from build123d import *

# Parameters (mm, degrees)
F0_W     = 33
F0_H     = 15
F1_DEPTH = 12
F2_W     = 31.2
F2_H     = 12.2
F3_DEPTH = 10
F4_W     = 30
F4_H     = 11
F5_DEPTH = 12.001


with BuildPart() as f1:
    # F0 (on Top) → F1 (new body)
    with BuildSketch(Plane.XY):
        with Locations((16.5, 7.5)):
            Rectangle(F0_W, F0_H)
    extrude(amount=F1_DEPTH)

    # F2 (on face) → F3 (cut)
    with BuildSketch(Plane.XY.offset(12)):
        with Locations((16.5, 7.5)):
            Rectangle(F2_W, F2_H)
    extrude(amount=-F3_DEPTH, mode=Mode.SUBTRACT)

    # F4 (on face) → F5 (cut, through all)
    with BuildSketch(Plane(origin=(0, 0, 0), x_dir=(1, 0, 0), z_dir=(0, 0, -1))):
        with Locations((16.5, -7.5)):
            Rectangle(F4_W, F4_H)
    extrude(amount=-F5_DEPTH, mode=Mode.SUBTRACT)


solid = f1.part
The model under review builds one solid part; all positions refer to its coordinate system, in mm. A direction names the side the tool comes from. Coordinates: 2 decimals unless noted, no trailing zeros. Write each loop counter-clockwise with the first axis right and the second up, starting at its lowest first coordinate (ties: lowest second). Pieces come first, ordered by that corner, then holes. Notation, with made-up numbers: (75.5, 52.5) - (106.5, 52.5) arc R25 cw to (106.5, 70.5) - close; hole circle Ø3 at (41.25, 68). An arc over 180 degrees is marked (long way). Answer as a JSON object with one key per item and string values. Group by question number.
1. Mouldability with a two-part tool opening along X and no side actions: class faces 1 (the face through (16, 13.6, 7)), 2 (the face through (18, 14, 12)), 3 (the face through (0, 7, 6)) as pulls with the +X half, pulls with the -X half, needs draft (parallel to the pull), parting line crosses it, or undercut.
2. Machinability: for faces 4 (the face through (16, 13, 1)), 5 (the face through (16, 0, 6)), 6 (the face through (32.1, 7, 7)), which of the approach directions +Z, -Z, +X, -X, +Y, -Y give a long, thin tool a straight path to every point of the face, cutting with its end or side? Answer none if there is none.
3. Add section B-B (y = 6.5). Give the boundary of the cut face in (x, z), plus the area to 3 significant figures.
4. Add section A-A (z = 3). Give the boundary of the cut face in (x, y).
5. To check wall thickness, follow probe 1 along Y at (x, z) = (30, 8.5); probe 2 along Y at (x, z) = (24, 1.75); probe 3 along X at (y, z) = (10, 9.5). State the ranges of each line that lie inside material, in increasing order.
6. Add section C-C (x = 25.5). Give the boundary of the cut face in (y, z), plus the area to 3 significant figures.
Findings:
{
 "1": {"face 1": "undercut", "face 2": "needs draft", "face 3": "pulls with the -X half"},
 "2": {"face 4": "+Z, -Z", "face 5": "+Z, -Z, +X, -X, -Y", "face 6": "+Z"},
 "3": {"outline": "(0, 0) - (1.5, 0) - (1.5, 2) - (0.9, 2) - (0.9, 12) - (0, 12) - close; (31.5, 0) - (33, 0) - (33, 12) - (32.1, 12) - (32.1, 2) - (31.5, 2) - close", "area": "24.0 mm²"},
 "4": {"outline": "(0, 0) - (33, 0) - (33, 15) - (0, 15) - close; hole (0.9, 1.4) - (32.1, 1.4) - (32.1, 13.6) - (0.9, 13.6) - close"},
 "5": {"probe 1": "0 to 1.4, 13.6 to 15", "probe 2": "0 to 2, 13 to 15", "probe 3": "0 to 0.9, 32.1 to 33"},
 "6": {"outline": "(0, 0) - (2, 0) - (2, 2) - (1.4, 2) - (1.4, 12) - (0, 12) - close; (13, 0) - (15, 0) - (15, 12) - (13.6, 12) - (13.6, 2) - (13, 2) - close", "area": "36.0 mm²"}
}
